Design review of the part built by this model. Coordinates are the model's own, in mm. Face numbers are marked on the shaded views. Round coordinates to 2 decimals unless told otherwise and drop trailing zeros. Order: outer loops, then holes, each group sorted by start corner. A loop starts at its lowest first (then second) coordinate and runs counter-clockwise, first axis right, second up. Notation, with made-up numbers: (53, 62) - (111, 62) arc R26 cw to (111, 82) - close; hole circle Ø1 at (16.25, 81.25). An arc over 180 degrees is marked (long way). Answer as a JSON object with one key per item and string values. Group by question number.
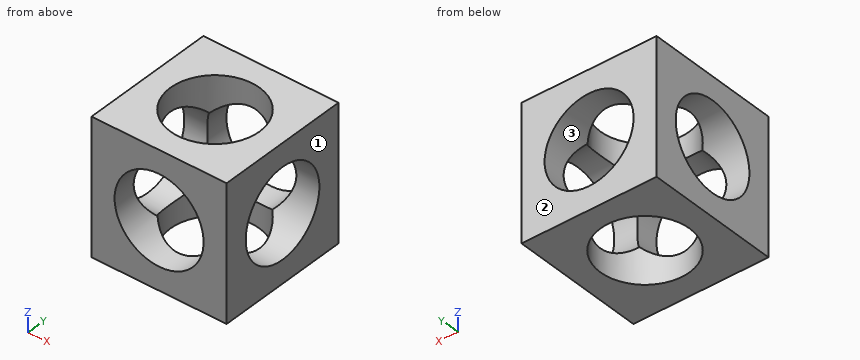
from build123d import *

# Parameters (mm, degrees)
ESQUISSE1_W                 = 22
ESQUISSE1_H                 = 22
BOSS_EXTRU_1_DEPTH          = 22
D_GAGEMENT_M131_D           = 14.5
D_GAGEMENT_M131_ON_FACE_2_D = 14.5
D_GAGEMENT_M131_ON_FACE_3_D = 14.5


with BuildPart() as part:
    # Esquisse1 → Boss.-Extru.1 (new body)
    with BuildSketch(Plane.XY):
        Rectangle(ESQUISSE1_W, ESQUISSE1_H)
    extrude(amount=BOSS_EXTRU_1_DEPTH)

    # Dégagement M131 (through all)
    with Locations(Plane(origin=(0, 11, 11), x_dir=(0, 0, 1), z_dir=(0, 1, 0))):
        with Locations((0, 0)):
            Hole(D_GAGEMENT_M131_D / 2)

    # Dégagement M131 on face 2 (through all)
    with Locations(Plane.XY.offset(22)):
        with Locations((0, 0)):
            Hole(D_GAGEMENT_M131_ON_FACE_2_D / 2)

    # Dégagement M131 on face 3 (through all)
    with Locations(Plane(origin=(11, 0, 11), x_dir=(0, 0, 1), z_dir=(1, 0, 0))):
        with Locations((0, 0)):
            Hole(D_GAGEMENT_M131_ON_FACE_3_D / 2)


solid = part.part
1. To check wall thickness, follow line 1 (X direction, y = 9.6, z = 11); line 2 (Z direction, x = 0, y = 9.05). State the ranges of each line that lie inside material, in increasing order. Write a range as from..to.
2. Clearance check with a flat-ended pin moving along its axis: P1, Ø6, axis at x = -1, y = -1.5, coming from the -Z side. State where the tip first meets the part, or that it passes through.
3. Take a section at D-D, the plane z = 20.5. Give the boundary of the cut face in (x, y).
4. Take a section at B-B, the plane x = 0. Give the boundary of the cut face in (y, z), then the cut area to 4 significant figures.
5. Mouldability with a two-part tool opening along X and no side actions: class the marked faces 1, 2 and 3 as pulls with the +X half, pulls with the -X half, needs draft (parallel to the pull), parting line crosses it, or undercut.
6. Take a section at A-A, the plane z = 11. Give the boundary of the cut face in (x, y).
7. Take a section at C-C, the plane y = -8. Give the boundary of the cut face in (x, z).
Response values:
{
 "1": {"line 1": "-11..-7.25, 7.25..11", "line 2": "0..3.75, 18.25..22"},
 "2": {"P1": "through"},
 "3": {"outline": "(-11, -11) - (11, -11) - (11, 11) - (-11, 11) - close; hole circle Ø14.5 at (0, 0)"},
 "4": {"outline": "(-11, 0) - (-7.25, 0) - (-7.25, 3.75) - (-11, 3.75) - close; (-11, 18.25) - (-7.25, 18.25) - (-7.25, 22) - (-11, 22) - close; (7.25, 0) - (11, 0) - (11, 3.75) - (7.25, 3.75) - close; (7.25, 18.25) - (11, 18.25) - (11, 22) - (7.25, 22) - close", "area": "56.25 mm2"},
 "5": {"face 1": "pulls with the +X half", "face 2": "needs draft", "face 3": "undercut"},
 "6": {"outline": "(-11, -11) - (-7.25, -11) - (-7.25, -7.25) - (-11, -7.25) - close; (-11, 7.25) - (-7.25, 7.25) - (-7.25, 11) - (-11, 11) - close; (7.25, -11) - (11, -11) - (11, -7.25) - (7.25, -7.25) - close; (7.25, 7.25) - (11, 7.25) - (11, 11) - (7.25, 11) - close"},
 "7": {"outline": "(-11, 0) - (11, 0) - (11, 22) - (-11, 22) - close; hole circle Ø14.5 at (0, 11)"}
}
